Input: part model. Units: mm. Frame: model coordinates. Face numbers are marked on the shaded views. A direction names the side the tool comes from. Round coordinates to 2 decimals unless told otherwise and drop trailing zeros. Write each loop counter-clockwise with the first axis right and the second up, starting at its lowest first coordinate (ties: lowest second). Pieces come first, ordered by that corner, then holes. Notation, with made-up numbers: (-38, -34) -> (-23, -34) arc R28 ccw to (-23, -5) -> close; hole circle Ø2 at (9.5, 73.5). An arc over 180 degrees is marked (long way). Use CSV: the item, a comma, the result in double quotes.
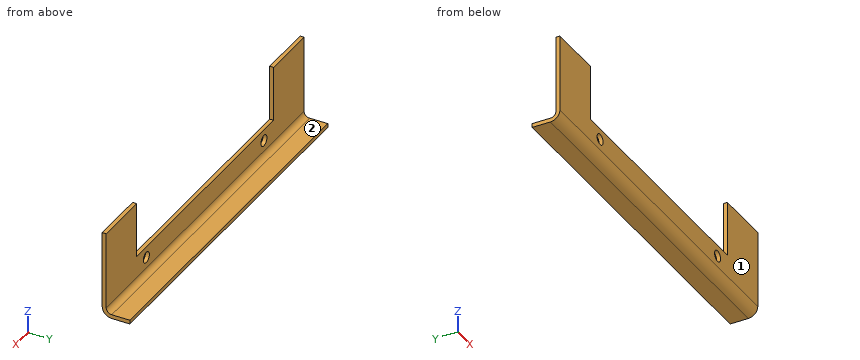
```python
from build123d import *

# Parameters (mm, degrees)
BASE_FLANGE1_DEPTH           = 0.91186
F_2_5MM_DOWEL_HOLE1_D        = 2.5
EDGE_FLANGE1_STRIP_W         = 6.18744
EDGE_FLANGE1_STRIP_H         = 0.91186
EDGE_FLANGE1_STRIP_CUT_DEPTH = 82.55
EDGE_FLANGE1_DEPTH           = 82.55


# Sheet-metal steps are written as plain solids
with BuildPart() as part:
    # Sketch1 → Base-Flange1 (new body)
    with BuildSketch(Plane(origin=(0, 0, 0), x_dir=(1, 0, 0), z_dir=(0, 1, 0))):
        Polygon((0, 0), (0, -19.05), (12.7, -19.05), (12.7, -6.35), (69.85, -6.35), (69.85, -19.05), (82.55, -19.05), (82.55, 0), align=None)
    extrude(amount=-BASE_FLANGE1_DEPTH)

    # Ø2.5mm Dowel Hole1 (through all)
    with Locations(Plane(origin=(0, -0.91186, 0), x_dir=(-1, 0, 0), z_dir=(0, -1, 0))):
        with Locations((-65.786, -3.81), (-16.764, -3.81)):
            Hole(F_2_5MM_DOWEL_HOLE1_D / 2)

    # Edge-Flange1 strip (across the edge) → Edge-Flange1 strip cut (cut)
    with BuildSketch(Plane.ZY.offset(-82.55)):
        with Locations((-1.82372, -0.45593)):
            Rectangle(EDGE_FLANGE1_STRIP_W, EDGE_FLANGE1_STRIP_H)
    extrude(amount=EDGE_FLANGE1_STRIP_CUT_DEPTH, mode=Mode.SUBTRACT)

    # Edge-Flange1 section (across the edge) → Edge-Flange1 (add)
    with BuildSketch(Plane.ZY.offset(-82.55)):
        with BuildLine():
            Line((-0.91186, 1.27), (-0.91186, 5.43814))
            Line((-0.91186, 5.43814), (0, 5.43814))
            Line((0, 5.43814), (0, 1.27))
            ThreePointArc((0, 1.27), (0.371974388, 0.371974388), (1.27, 0))
            Line((1.27, 0), (1.27, -0.91186))
            ThreePointArc((1.27, -0.91186), (-0.272808002, -0.272808002), (-0.91186, 1.27))
        make_face()
    extrude(amount=EDGE_FLANGE1_DEPTH)


solid = part.part
```
Item 1: First-contact query: pin 1 Ø1.3 at (x, y) = (29, 2.5) entering from +Z; pin 2 Ø3 at (x, z) = (65.786, 3.81) entering from +Y; pin 3 Ø0.5 at (x, y) = (33, -0.5) entering from +Z. Flat tips, straight axial feed; report the tip coordinate or a pass-through.
Worked answers:
pin 1,"stops at z = 0"
pin 2,"stops at y = 0"
pin 3,"stops at z = 6.35"
Item 2: Section query C-C on z = 3.81. Return the cut outline in (x, y), plus the area to 3 significant figures.
Worked answers:
outline,"(0, -0.91) -> (15.51, -0.91) -> (15.51, 0) -> (0, 0) -> close; (18.01, -0.91) -> (64.54, -0.91) -> (64.54, 0) -> (18.01, 0) -> close; (67.04, -0.91) -> (82.55, -0.91) -> (82.55, 0) -> (67.04, 0) -> close"
area,"70.7 mm²"
Item 3: Section query D-D on y = 2. Return the cut outline in (x, z), plus the area to 3 significant figures.
Worked answers:
outline,"(0, -0.91) -> (82.55, -0.91) -> (82.55, 0) -> (0, 0) -> close"
area,"75.3 mm²"
Item 4: Line query: line 1 (Z direction, x = 39, y = 2.5); line 2 (Z direction, x = 4, y = -0.25). Output: solid intervals per line, ascending.
Worked answers:
line 1,"z = -0.91 to 0"
line 2,"z = -0.3 to 19.05"
Item 5: Section query B-B on x = 34. Return the cut outline in (y, z), plus the area to 3 significant figures.
Worked answers:
outline,"(-0.91, 1.27) arc R2.18 ccw to (1.27, -0.91) -> (5.44, -0.91) -> (5.44, 0) -> (1.27, 0) arc R1.27 cw to (0, 1.27) -> (0, 6.35) -> (-0.91, 6.35) -> close"
area,"10.9 mm²"
Item 6: Section query A-A on z = 16.25. Return the cut outline in (x, y), plus the area to 3 significant figures.
Worked answers:
outline,"(0, -0.91) -> (12.7, -0.91) -> (12.7, 0) -> (0, 0) -> close; (69.85, -0.91) -> (82.55, -0.91) -> (82.55, 0) -> (69.85, 0) -> close"
area,"23.2 mm²"
Item 7: Set-up query: the marked faces 1 and 2. Return all of +Z, -Z, +X, -X, +Y, -Y with unobstructed straight access to the full face (end or side cutting, diameter ignored); none if empty.
Worked answers:
face 1,"+Z, -Z, +X, -X, -Y"
face 2,"+Z, +X, -X, +Y"
